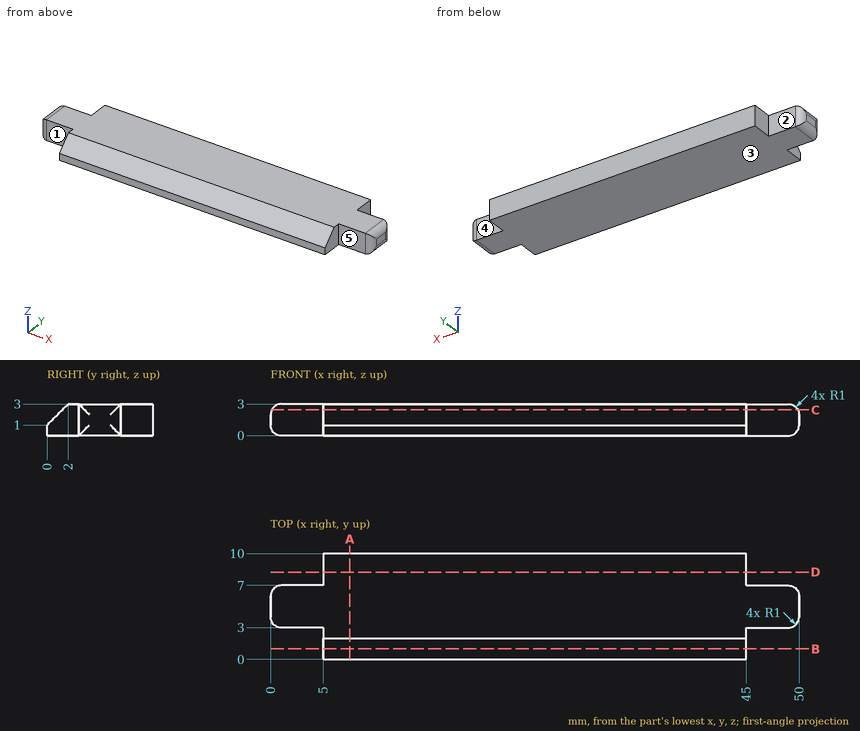
Here's the drawing with two shaded views (mm, measured from the low corner). I have some questions. A direction names the side the tool comes from. Round coordinates to 2 decimals unless told otherwise and drop trailing zeros. Loops run counter-clockwise (first coordinate to the right, second up) from the corner with the lowest first, then second, coordinate; pieces in that order, holes last. Notation, with made-up numbers: M -24,-5 L 14,-5 A30 ccw 14,23 Z; hole C -35.5,25 d5. An arc over 180 degrees is marked long. Answer as CSV lines item,"result".
1) For pin 1 Ø0.9 at (y, z) = (9, 1) entering from -X; pin 2 Ø0.9 at (x, z) = (46.5, 2) entering from +Y; pin 3 Ø1.5 at (y, z) = (7.5, 1) entering from -X, each with a flat end and sliding along its axis, tell me the tip position at first contact or that it passes through.
From the geometry:
pin 1,"x = 5"
pin 2,"y = 7"
pin 3,"x = 0.34"
2) Imagine slicing it at C-C on z = 2.45. List the corners of the cut face in (x, y) for me.
From the geometry:
outline,"M 0.11,3.55 A1 ccw 1,3 L 5,3 L 5,1.45 L 45,1.45 L 45,3 L 49,3 A1 ccw 49.89,3.55 L 49.89,6.45 A1 ccw 49,7 L 45,7 L 45,10 L 5,10 L 5,7 L 1,7 A1 ccw 0.11,6.45 Z"
3) Which directions (+Z, -Z, +X, -X, +Y, -Y) give clear straight access to the entire face, cutting with the end or side of a thin tool? Please do the marked faces 1, 2, 3, 4 and 5.
From the geometry:
face 1,"+Z, -Z, -X, -Y"
face 2,"+Z, -Z, -X, +Y"
face 3,"-Z, +X, -X, +Y, -Y"
face 4,"+Z, -Z, +X, +Y"
face 5,"+Z, -Z, +X, -Y"
4) Imagine slicing it at B-B on y = 1. List the corners of the cut face in (x, z) for me, and give its area (3 significant figures).
From the geometry:
outline,"M 5,0 L 45,0 L 45,2 L 5,2 Z"
area,"80.0 mm^2"
5) If I drill on probe 1 along X at (y, z) = (7.25, 0.6); probe 2 along Y at (x, z) = (4, 0.75); probe 3 along Z at (x, y) = (7, 1), over which ranges is the centre line in solid material (lowest first)?
From the geometry:
probe 1,"5 to 45"
probe 2,"3 to 7"
probe 3,"0 to 2"
6) Imagine slicing it at D-D on y = 8.25. List the corners of the cut face in (x, z) for me.
From the geometry:
outline,"M 5,0 L 45,0 L 45,3 L 5,3 Z"
7) Imagine slicing it at A-A on x = 7.5. List the corners of the cut face in (y, z) for me.
From the geometry:
outline,"M 0,0 L 10,0 L 10,3 L 2,3 L 0,1 Z"
